Work out the finished part from the listing and answer in its coordinate system (mm). Face numbers are marked on the shaded views. Give positions to 0.01 mm unless a question says otherwise; leave off trailing zeros. Order: outer loops, then holes, each group sorted by start corner. A loop starts at its lowest first (then second) coordinate and runs counter-clockwise, first axis right, second up. Notation, with made-up numbers: (11, -19.5) -> (67, -19.5) arc R16 ccw to (67, -10.5) -> close; hole circle Ø7 at (0.5, -37.5). An arc over 180 degrees is marked (long way). Answer as CSV lines item,"result". Start each with the question number.
1. A cutting plane is placed at B-B (z = 1.3). Give the vertices of the cut face in (x, y), then the cut area to 3 significant figures.
2. A cutting plane is placed at A-A (y = 0). Give the vertices of the cut face in (x, z) (3 decimals).
3. A flat-ended cylindrical pin translates along its axis: pin 1 (2.5 mm diameter, centred on x = 7.76, y = 0, fed in from +Z). Find the tip coordinate at first contact, or state that the pin passes through.
4. A cutting plane is placed at C-C (x = -7.75). Give the vertices of the cut face in (y, z) (3 decimals).
5. For a pull along X with two mould halves and no side action, classify the marked faces 1, 2 and 3 as released by +X, released by -X, zero draft, split by the parting line, or undercut.
6. Find the intervals of material crossed by L1, parallel to X at y = 0.25, z = 0.3; L2, parallel to Y at x = 7.5, z = 1.4; L3, parallel to Y at x = -9.25, z = 1.55, in increasing order.
from build123d import *

# Parameters (mm, degrees)
SKETCH1_W           = 25.5
SKETCH1_H           = 13
BOSS_EXTRUDE1_DEPTH = 3.175
SKETCH2_R           = 2
CUT_EXTRUDE1_DEPTH  = 15.788505467


with BuildPart() as part:
    # Sketch1 → Boss-Extrude1 (new body)
    with BuildSketch(Plane.XY):
        with Locations((0.009203008, -0.269195489)):
            Rectangle(SKETCH1_W, SKETCH1_H)
    extrude(amount=BOSS_EXTRUDE1_DEPTH)

    # Sketch2 → Cut-Extrude1 (cut, through all)
    with BuildSketch(Plane(origin=(0, 0, 0), x_dir=(-1, 0, 0), z_dir=(0, 0, -1))):
        with Locations((-7.759203008, 0)):
            Circle(SKETCH2_R)
        with Locations((7.740796992, 0)):
            Circle(SKETCH2_R)
    extrude(amount=-CUT_EXTRUDE1_DEPTH, mode=Mode.SUBTRACT)


solid = part.part
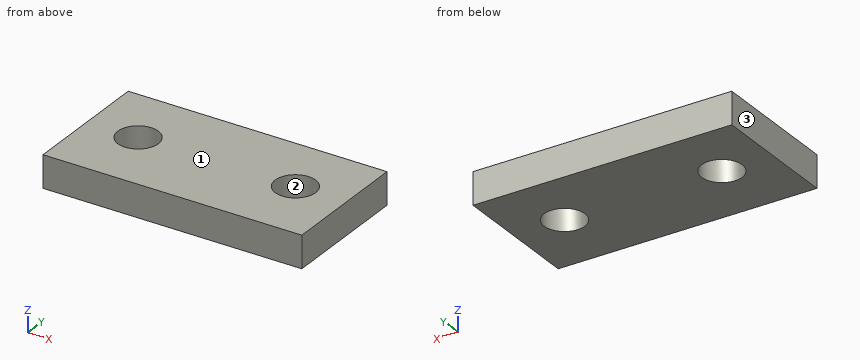
Answer sheet:
1,outline,"(-12.74, -6.77) -> (12.76, -6.77) -> (12.76, 6.23) -> (-12.74, 6.23) -> close; hole circle Ø4 at (-7.74, 0); hole circle Ø4 at (7.76, 0)"
1,area,"306 mm^2"
2,outline,"(-12.741, 0) -> (-9.741, 0) -> (-9.741, 3.175) -> (-12.741, 3.175) -> close; (-5.741, 0) -> (5.759, 0) -> (5.759, 3.175) -> (-5.741, 3.175) -> close; (9.759, 0) -> (12.759, 0) -> (12.759, 3.175) -> (9.759, 3.175) -> close"
3,pin 1,"passes through"
4,outline,"(-6.769, 0) -> (-2, 0) -> (-2, 3.175) -> (-6.769, 3.175) -> close; (2, 0) -> (6.231, 0) -> (6.231, 3.175) -> (2, 3.175) -> close"
5,face 1,"zero draft"
5,face 2,"undercut"
5,face 3,"released by -X"
6,L1,"x = -12.74 to -9.73, -5.76 to 5.77, 9.74 to 12.76"
6,L2,"y = -6.77 to -1.98, 1.98 to 6.23"
6,L3,"y = -6.77 to -1.31, 1.31 to 6.23"
